Geometry: see drawing. Coordinates: mm, zero at the bounding-box minimum. A direction names the side the tool comes from. Give positions to 0.01 mm unless a question says otherwise; leave off trailing zeros. Write each loop counter-clockwise with the first axis right and the second up, starting at its lowest first coordinate (ties: lowest second). Pieces come first, ordered by that corner, then holes. Notation, with made-up numbers: (76.25, 3) - (129.25, 3) arc R18 cw to (129.25, 7) - close; hole circle Ø6 at (34.5, 0). An arc over 180 degrees is marked (long way). Use a Markdown table: item, result. Add a question column.
1. Pin query (flat end, axial travel): pin 1 (1 mm diameter, centred on x = 20.5, z = 22, fed in from +Y); pin 2 (24 mm diameter, centred on x = 20.5, y = 20.5, fed in from -Z); pin 3 (3 mm diameter, centred on x = 18.5, z = 21.5, fed in from -Y); pin 4 (1 mm diameter, centred on x = 7, y = 31.5, fed in from +Z). Return the tip coordinate at first contact, or that it passes through.
2. Section query A-A, the plane x = 20.5. Return loops of the section in (y, z), plus the area to 3 significant figures.
3. Mould query, pull axis Y, two halves, no side actions, for the marked faces 3 and 4. Classes: released by +Y, released by -Y, zero draft, split by the parting line, or undercut.
4. Section query C-C, the plane z = 17. Return loops of the section in (x, y).
5. Set-up query: the marked faces 1 and 2. Return all of +Z, -Z, +X, -X, +Y, -Y with unobstructed straight access to the full face (end or side cutting, diameter ignored); none if empty.
6. Section query D-D, the plane z = 4. Return loops of the section in (x, y), plus the area to 3 significant figures.
7. Material intervals for probe 1 along Y at (x, z) = (20.5, 4.25); probe 2 along Y at (x, z) = (20.5, 10.5); probe 3 along X at (y, z) = (12, 17.5), sorted ascending.
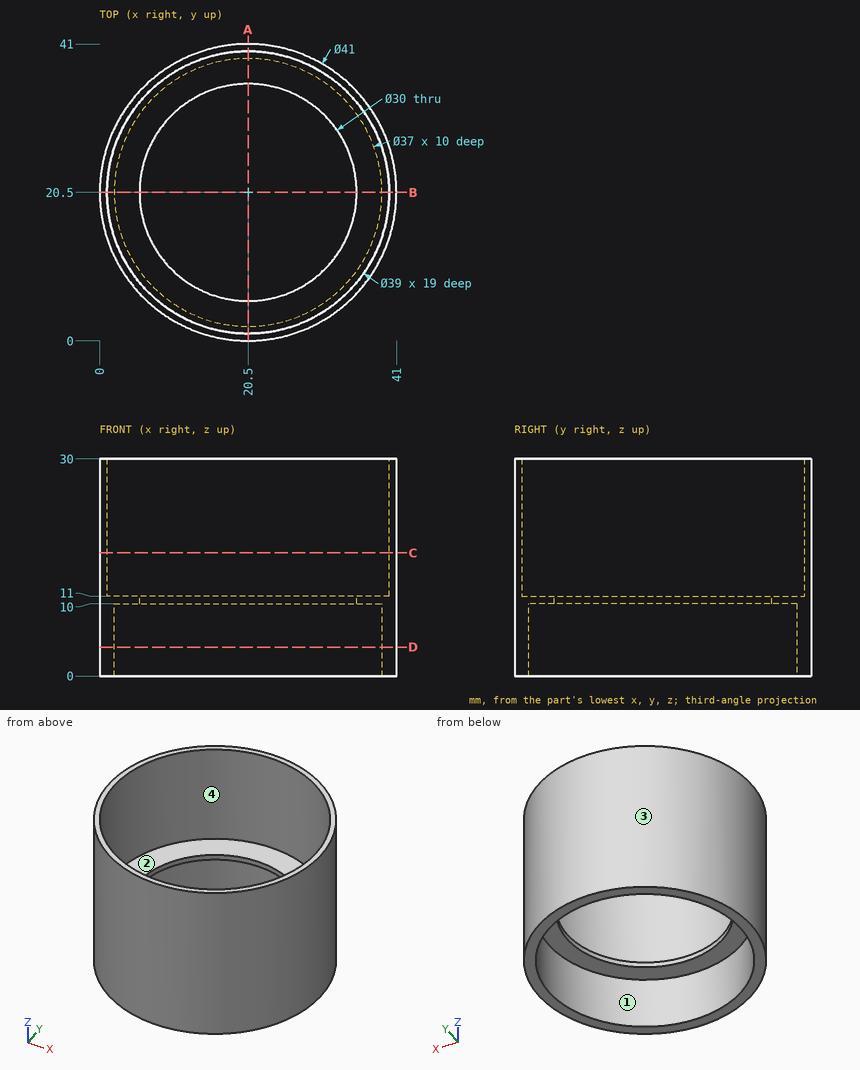
Result sheet:
| question | item | result |
|---|---|---|
| 1 | pin 1 | stops at y = 41 |
| 1 | pin 2 | passes through |
| 1 | pin 3 | stops at y = 0.01 |
| 1 | pin 4 | stops at z = 11 |
| 2 | outline | (0, 0) - (2, 0) - (2, 10) - (5.5, 10) - (5.5, 11) - (1, 11) - (1, 30) - (0, 30) - close; (35.5, 10) - (39, 10) - (39, 0) - (41, 0) - (41, 30) - (40, 30) - (40, 11) - (35.5, 11) - close |
| 2 | area | 89.0 mm² |
| 3 | face 3 | split by the parting line |
| 3 | face 4 | undercut |
| 4 | outline | circle Ø41 at (20.5, 20.5); hole circle Ø39 at (20.5, 20.5) |
| 5 | face 1 | -Z |
| 5 | face 2 | +Z |
| 6 | outline | circle Ø41 at (20.5, 20.5); hole circle Ø37 at (20.5, 20.5) |
| 6 | area | 245 mm² |
| 7 | probe 1 | y = 0 to 2, 39 to 41 |
| 7 | probe 2 | y = 0 to 5.5, 35.5 to 41 |
| 7 | probe 3 | x = 1.85 to 2.95, 38.05 to 39.15 |
